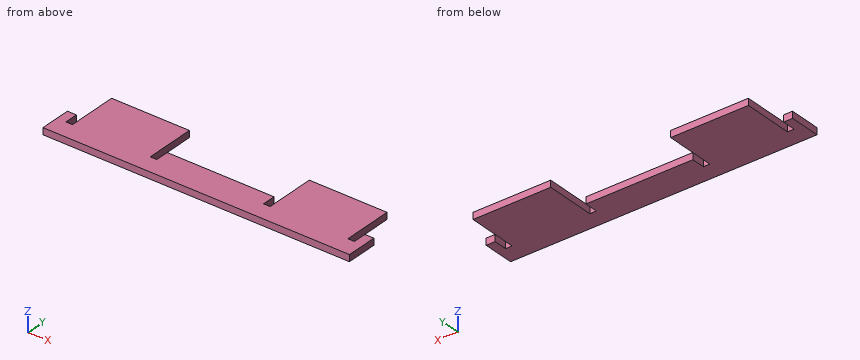
Autodesk Inventor part; units mm, degrees
ref_plane "YZ Plane" through (0, 0, 0) normal (1, 0, 0) x (0, 1, 0)
ref_plane "XZ Plane" through (0, 0, 0) normal (0, 1, 0) x (-1, 0, 0)
ref_plane "XY Plane" through (0, 0, 0) normal (0, 0, 1) x (1, 0, 0)
sketch "草圖1" plane through (0, 0, 0) normal (0, 0, 1) x (1, 0, 0)
  line L0 (0, 0) -> (124, 0)
  line L1 (124, 0) -> (124, -14) construction
  line L2 (124, -14) -> (0, -14)
  line L3 (0, -14) -> (0, 0) construction
  line L4 (35, 0) -> (37.95, 0)
  line L5 (37.95, 0) -> (37.95, -6)
  line L6 (37.95, -6) -> (35, -6)
  line L7 (35, -6) -> (35, 0)
  line L8 (89, 0) -> (86.05, 0)
  line L9 (86.05, 0) -> (86.05, -6)
  line L10 (86.05, -6) -> (89, -6)
  line L11 (89, -6) -> (89, 0)
  line L12 (131, -14) -> (126.95, -14)
  line L13 (124, 0) -> (131, 0)
  line L14 (131, 0) -> (131, -14)
  line L15 (126.95, -14) -> (126.95, -6)
  line L16 (126.95, -6) -> (124, -6)
  line L17 (0, 0) -> (-7, 0)
  line L18 (-7, 0) -> (-7, -14)
  line L19 (-7, -14) -> (-2.95, -14)
  line L20 (0, -14) -> (0, 0) construction
  line L21 (-2.95, -14) -> (-2.95, -6)
  line L22 (-2.95, -6) -> (0, -6)
  line L23 (0, -6) -> (0, -14)
  line L24 (124, -6) -> (124, -14)
  line L25 (124, -14) -> (126.95, -14)
  line L26 (124, -6) -> (126.95, -6)
  line L27 (126.95, -6) -> (126.95, 0)
  line L28 (126.95, 0) -> (124, 0)
  line L29 (124, 0) -> (124, -6)
  line L30 (-2.95, -14) -> (0, -14)
  line L31 (-2.95, -6) -> (0, -6)
  line L32 (0, -6) -> (0, 0)
  line L33 (0, 0) -> (-2.95, 0)
  line L34 (-2.95, 0) -> (-2.95, -6)
  point P0 (0, -15.5)
  point P1 (0, -6)
  point P2 (0, -14)
  dimension "d0" = 124
  dimension "d1" = 35
  dimension "d3" = 2.95
  dimension "d4" = 2.95
  dimension "d10" = 8
  dimension "d16" = 6
  dimension "d17" = 35
  dimension "d18" = 2.95
  dimension "d21" = 7
  dimension "d22" = 2.95
  dimension "d24" = 7
  dimension "d29" = 6
  dimension "d30" = 6
extrude "擠出1" add sketch "草圖1" along normal blind 3 contours L0 L7 L6 L5 L9 L10 L11 L29 L24 L2 L23 L32 | L34 L21 L19 L18 L17 | L23 L30 L21 L22 | L24 L16 L15 L25 | L15 L27 L13 L14 L12
move faces "移動2" translate (0, 16.5, 0) faces at (23.3333, 0, 1) (112.3333, 0, 1)
properties part number "chassis_1_7"
Here's how the part is built. I have some questions about the finished solid (model axes, mm). Give positions to 0.01 mm unless a question says otherwise; leave off trailing zeros. Order: outer loops, then holes, each group sorted by start corner. A loop starts at its lowest first (then second) coordinate and runs counter-clockwise, first axis right, second up. Notation, with made-up numbers: M -6.75,13.5 L 0.25,13.5 A33 ccw 0.25,41.5 Z; hole C 42.25,49 d11. An arc over 180 degrees is marked long. Answer as a JSON object with one key per item and string values. Group by question number.
1) Please list where these lines run through material, in increasing order: L1, parallel to X at y = -4, z = 0.4; L2, parallel to X at y = 11.5, z = 0.55; L3, parallel to Y at x = 69, z = 2.2. Write a range as [from, to].
2) Suppose I cut it at D-D, the plane x = 75.5. Write out the boundary of the cut face in (y, z), plus the area to 3 significant figures.
3) Suppose I cut it at B-B, the plane y = 3.5. Write out the boundary of the cut face in (x, z).
4) Suppose I cut it at C-C, the plane z = 0.65. Write out the boundary of the cut face in (x, y).
5) I'm going to push flat-ended pins straight in: pin 1 Ø1.5 at (x, z) = (-1.5, 1.5) entering from +Y; pin 2 Ø0.9 at (y, z) = (2, 2) entering from +X; pin 3 Ø0.9 at (x, z) = (128, 1) entering from +Y. Where does each tip first touch, or does it pass through?
6) Suppose I cut it at A-A, the plane y = -2. Write out the boundary of the cut face in (x, z), plus the area to 3 significant figures.
Results found:
{
 "1": {"L1": "[-7, -2.95], [0, 35], [37.95, 86.05], [89, 124], [126.95, 131]", "L2": "[0, 35], [89, 124]", "L3": "[-14, 0]"},
 "2": {"outline": "M -14,0 L 0,0 L 0,3 L -14,3 Z", "area": "42.0 mm²"},
 "3": {"outline": "M 0,0 L 35,0 L 35,3 L 0,3 Z; M 89,0 L 124,0 L 124,3 L 89,3 Z"},
 "4": {"outline": "M -7,-14 L 131,-14 L 131,0 L 126.95,0 L 126.95,-6 L 124,-6 L 124,16.5 L 89,16.5 L 89,-6 L 86.05,-6 L 86.05,0 L 37.95,0 L 37.95,-6 L 35,-6 L 35,16.5 L 0,16.5 L 0,-6 L -2.95,-6 L -2.95,0 L -7,0 Z"},
 "5": {"pin 1": "y = -6", "pin 2": "x = 124", "pin 3": "y = 0"},
 "6": {"outline": "M -7,0 L -2.95,0 L -2.95,3 L -7,3 Z; M 0,0 L 35,0 L 35,3 L 0,3 Z; M 37.95,0 L 86.05,0 L 86.05,3 L 37.95,3 Z; M 89,0 L 124,0 L 124,3 L 89,3 Z; M 126.95,0 L 131,0 L 131,3 L 126.95,3 Z", "area": "379 mm²"}
}
